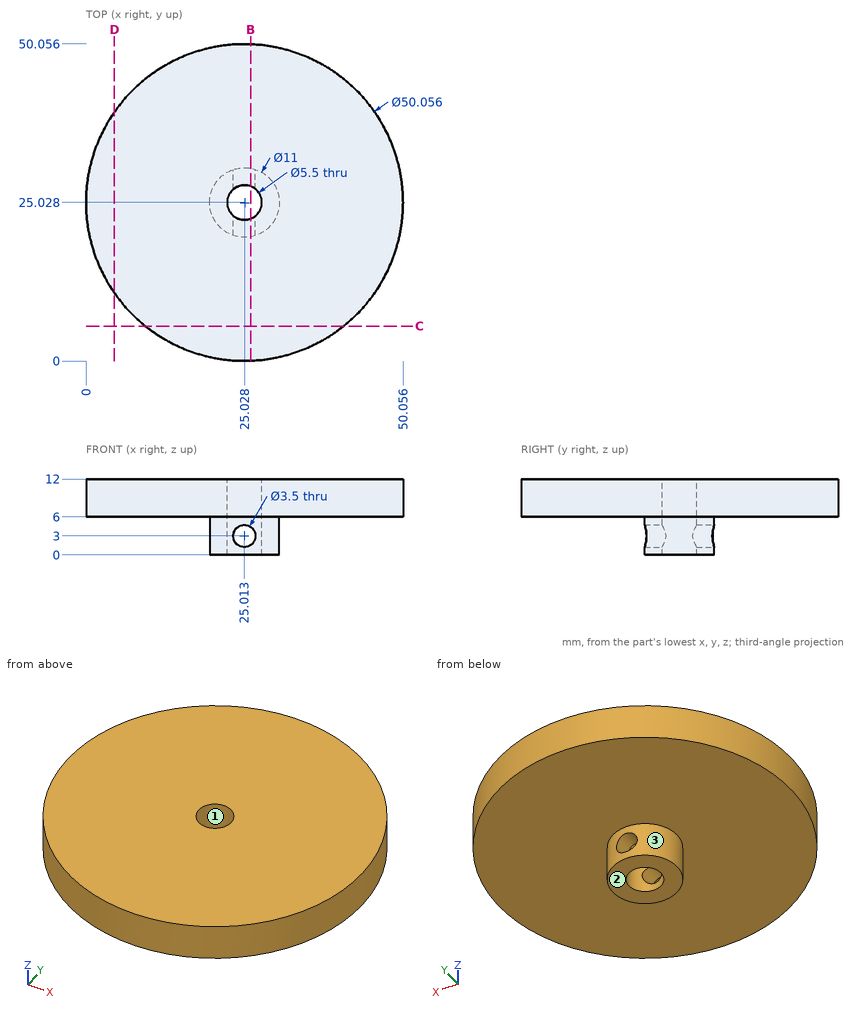
Answer from the drawing. Dimensions are ordinates in mm from the lowest x, y and z of the part. Coordinates: 2 decimals unless noted, no trailing zeros. Loops run counter-clockwise (first coordinate to the right, second up) from the corner with the lowest first, then second, coordinate; pieces in that order, holes last.
Q1. The part is cut by section B-B on x = 26. Write down the section's boundary in (y, z) (1 decimal), and give its area (3 significant figures).
Q2. Each of these flat-tipped pins is pushed along its axis until it touches: pin 1 Ø2 at (x, z) = (19, 6.5) entering from +Y (1 decimal); pin 2 Ø3 at (x, z) = (25.01, 3) entering from +Y; pin 3 Ø4.5 at (x, z) = (25.01, 3) entering from -Y; pin 4 Ø2 at (y, z) = (21.5, 8.5) entering from +X. Where does it stop, or does it pass through?
Q3. Consider probe 1 along Z at (x, y) = (43, 21.5); probe 2 along X at (y, z) = (21, 4.5) (1 decimal); probe 3 along Y at (x, z) = (25.5, 5). Determine where each line is inside the solid, lowest interval first.
Q4. The mould has two halves that part along Y. Classify the marked faces 1, 2 and 3: +Y half, -Y half, draft (parallel to the pull), parting line (faces both ways), or undercut.
Q5. The part is cut by section C-C on y = 5.5. Write down the section's boundary in (x, z).
Q6. The part is cut by section D-D on x = 4.5. Write down the section's boundary in (y, z) (1 decimal), and give its area (3 significant figures).
Results below:
1. outline: (0, 6) - (19.6, 6) - (19.6, 4.4) - (22.5, 4.4) - (22.5, 12) - (0, 12) - close; (19.6, 0) - (22.5, 0) - (22.5, 1.6) - (19.6, 1.6) - close; (27.6, 0) - (30.4, 0) - (30.4, 1.6) - (27.6, 1.6) - close; (27.6, 4.4) - (30.4, 4.4) - (30.4, 6) - (50, 6) - (50, 12) - (27.6, 12) - close
1. area: 287 mm2
2. pin 1: stops at y = 49.5
2. pin 2: passes through
2. pin 3: stops at y = 19.53
2. pin 4: stops at x = 49.93
3. probe 1: z = 6 to 12
3. probe 2: x = 21.3 to 24.1, 25.9 to 28.8
3. probe 3: y = 19.55 to 22.32, 27.74 to 30.51
4. face 1: undercut
4. face 2: draft
4. face 3: parting line
5. outline: (9.37, 6) - (40.68, 6) - (40.68, 12) - (9.37, 12) - close
6. outline: (10.7, 6) - (39.3, 6) - (39.3, 12) - (10.7, 12) - close
6. area: 172 mm2
